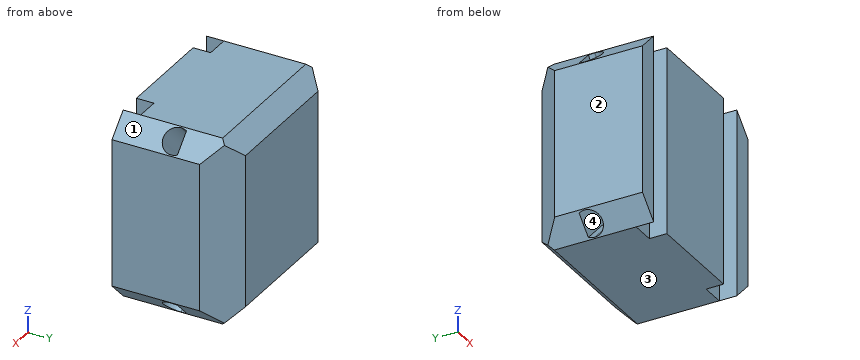
from build123d import *

# Parameters (mm, degrees)
SKETCH1_W                                = 160
SKETCH1_H                                = 160
BOSS_EXTRUDE1_DEPTH                      = 100
CHAMFER1_SIZE                            = 25
CHAMFER2_SIZE                            = 17
CHAMFER3_SIZE                            = 15
CUT_EXTRUDE1_DEPTH                       = 50
SKETCH3_W                                = 20
SKETCH3_H                                = 160
CUT_EXTRUDE2_DEPTH                       = 15
MIRROR1_AT_THE_SECOND_PLANE_COPY_1_DEPTH = 50


with BuildPart() as part:
    # Sketch1 → Boss-Extrude1 (new body)
    with BuildSketch(Plane(origin=(0, 0, 0), x_dir=(1, 0, 0), z_dir=(0, 1, 0))):
        with Locations((-95.343060511, -3.92868134)):
            Rectangle(SKETCH1_W, SKETCH1_H)
    extrude(amount=BOSS_EXTRUDE1_DEPTH)

    # Chamfer1
    chamfer1_edges = [part.edges().sort_by_distance(p)[0] for p in [
        (-15.343060511, 100, 3.92868134),
        (-175.343060511, 100, 3.92868134),
    ]]
    chamfer(chamfer1_edges, length=CHAMFER1_SIZE)

    # Chamfer2
    chamfer2_edges = [part.edges().sort_by_distance(p)[0] for p in [
        (-15.343060511, 37.5, 83.92868134),
        (-175.343060511, 37.5, 83.92868134),
        (-175.343060511, 37.5, -76.07131866),
        (-15.343060511, 37.5, -76.07131866),
    ]]
    chamfer(chamfer2_edges, length=CHAMFER2_SIZE)

    # Chamfer3
    chamfer3_edges = [part.edges().sort_by_distance(p)[0] for p in [
        (-95.343060511, 100, 83.92868134),
        (-95.343060511, 100, -76.07131866),
    ]]
    chamfer(chamfer3_edges, length=CHAMFER3_SIZE)

    # Sketch2 → Cut-Extrude1 (cut)
    with BuildSketch(Plane(origin=(21.864129074, 0, -21.864129074), x_dir=(-0.7071067811865471, 0, -0.7071067811865479), z_dir=(0.7071067811865479, 0, -0.7071067811865471))):
        with BuildLine():
            ThreePointArc((75.669890857, 50), (75.36515964, 52.571230378), (74.467849828, 55))
            Line((74.467849828, 55), (64.669890857, 55))
            Line((64.669890857, 55), (54.871931886, 55))
            ThreePointArc((54.871931886, 55), (62.098660479, 39.304731217), (75.669890857, 50))
        make_face()
    cut_extrude1 = extrude(amount=-CUT_EXTRUDE1_DEPTH, mode=Mode.SUBTRACT)

    # Sketch3 → Cut-Extrude2 (cut)
    with BuildSketch(Plane.XZ):
        with Locations((-148.343060511, 3.92868134)):
            Rectangle(SKETCH3_W, SKETCH3_H)
        with Locations((-42.343060511, 3.92868134)):
            Rectangle(SKETCH3_W, SKETCH3_H)
    extrude(amount=-CUT_EXTRUDE2_DEPTH, mode=Mode.SUBTRACT)

    # Mirror1: Cut-Extrude1 across plane
    add(cut_extrude1.mirror(Plane(origin=(0, 0, 3.92868134), x_dir=(1, 0, 0), z_dir=(0, 0, -1))), mode=Mode.SUBTRACT)

    # Mirror1 at the second plane: Cut-Extrude1 across plane
    add(cut_extrude1.mirror(Plane.ZY.offset(95.343060511)), mode=Mode.SUBTRACT)

    # Mirror1 at the second plane copy 1 sketc → Mirror1 at the second plane copy 1 (cut)
    with BuildSketch(Plane(origin=(-212.550250097, 0, 29.721491754), x_dir=(0.7071067811865474, 0, 0.7071067811865477), z_dir=(-0.7071067811865477, 0, 0.7071067811865474))):
        with BuildLine():
            ThreePointArc((75.669890857, 50), (75.36515964, 52.571230378), (74.467849828, 55))
            Line((74.467849828, 55), (64.669890857, 55))
            Line((64.669890857, 55), (54.871931886, 55))
            ThreePointArc((54.871931886, 55), (62.098660479, 39.304731217), (75.669890857, 50))
        make_face()
    extrude(amount=-MIRROR1_AT_THE_SECOND_PLANE_COPY_1_DEPTH, mode=Mode.SUBTRACT)


solid = part.part
Geometry check sheet. Reference: the model listing, model coordinates, mm. Face numbers are marked on the shaded views. Round coordinates to 2 decimals unless told otherwise and drop trailing zeros. Order: outer loops, then holes, each group sorted by start corner. A loop starts at its lowest first (then second) coordinate and runs counter-clockwise, first axis right, second up. Notation, with made-up numbers: M 3,-11 L 20,-11 A10 cw 20,5 Z; hole C 76.5,-15 d10. An arc over 180 degrees is marked long. Answer in a Markdown table with one row per item. Add a question column.
Item 1: Sectioned sample at A-A, the plane y = 60. Enter the section's corners in (x, z), plus the area to 3 significant figures.
Item 2: Sectioned sample at C-C, the plane z = -34. State how many separate pieces and enclosed holes the cut face has, plus the area to 3 significant figures.
Item 3: Draft check along X on the marked faces 1, 2, 3 and 4. Enter one of: released by +X, released by -X, zero draft, split by the parting line, or undercut.
Item 4: Material ranges on L1, parallel to Z at x = -58.5, y = 49; L2, parallel to X at y = 49, z = -43.5; L3, parallel to X at y = 43, z = -27, recorded low to high. Write a range as [from, to].
Item 5: Sectioned sample at B-B, the plane z = -2. Enter the section's corners in (x, y), plus the area to 3 significant figures.
Item 6: Depth check by flat-ended pin: pin 1 Ø15 at (x, z) = (-41.5, 66.5) entering from -Y; pin 2 Ø2 at (x, y) = (-97, 87.5) entering from +Z. Enter the tip coordinate at first touch or a pass-through.
Filled in:
| question | item | result |
|---|---|---|
| 1 | outline | M -175.34,-59.07 L -158.34,-76.07 L -32.34,-76.07 L -15.34,-59.07 L -15.34,66.93 L -32.34,83.93 L -158.34,83.93 L -175.34,66.93 Z |
| 1 | area | 25,000 mm² |
| 2 | separate pieces | 1 |
| 2 | enclosed holes | 2 |
| 2 | area | 14,200 mm² |
| 3 | face 1 | released by +X |
| 3 | face 2 | released by -X |
| 3 | face 3 | zero draft |
| 3 | face 4 | undercut |
| 4 | L1 | z = [-76.07, -48.45], [-31.52, 39.37], [56.31, 83.93] |
| 4 | L2 | x = [-175.34, -158.22], [-127.24, -63.45], [-32.47, -15.34] |
| 4 | L3 | x = [-175.34, -138.23], [-136.7, -53.98], [-52.46, -15.34] |
| 5 | outline | M -175.34,0 L -158.34,0 L -158.34,15 L -138.34,15 L -138.34,0 L -52.34,0 L -52.34,15 L -32.34,15 L -32.34,0 L -15.34,0 L -15.34,75 L -40.34,100 L -150.34,100 L -175.34,75 Z |
| 5 | area | 14,800 mm² |
| 6 | pin 1 | stops at y = 15 |
| 6 | pin 2 | stops at z = 82.43 |
